from build123d import *

# Parameters (mm, degrees)
SKETCH1_R         = 9.5
SKETCH1_R_2       = 8
EXTRUDE1_DEPTH    = 1.5
SKETCH2_R         = 10.5
SKETCH2_R_2       = 8
EXTRUDE2_DEPTH    = 1.5
EXTRUDE3_START    = 6.5
SKETCH3_R         = 9.5
EXTRUDE3_DEPTH    = 6.5
EXTRUDE4_START    = 1.5
SKETCH4_R         = 9.5
SKETCH4_R_2       = 5
EXTRUDE4_DEPTH    = 1.5
SKETCH5_R         = 5
EXTRUDE5_DEPTH    = 19.479718613
SKETCH6_R         = 0.75
EXTRUDE6_DEPTH    = 18.628102564
CIRPATTERN1_COUNT = 4
EXTRUDE7_START    = 10
SKETCH7_R         = 6.5
SKETCH7_R_2       = 5
EXTRUDE7_DEPTH    = 10
SKETCH8_R         = 6.5
SKETCH8_W         = 5
SKETCH8_H         = 5
EXTRUDE8_DEPTH    = 1.5


with BuildPart() as part:
    # Sketch1 → Extrude1 (new body)
    with BuildSketch(Plane.XY):
        Circle(SKETCH1_R)
        Circle(SKETCH1_R_2, mode=Mode.SUBTRACT)
    extrude(amount=EXTRUDE1_DEPTH)

    # Sketch2 → Extrude2 (add)
    with BuildSketch(Plane.XY.offset(1.5)):
        Circle(SKETCH2_R)
        Circle(SKETCH2_R_2, mode=Mode.SUBTRACT)
    extrude(amount=EXTRUDE2_DEPTH)

    # Sketch3 → Extrude3 (add)
    with BuildSketch(Plane(origin=(0, 0, 0), x_dir=(-1, 0, 0), z_dir=(0, 0, -1)).offset(EXTRUDE3_START)):
        Circle(SKETCH3_R)
        with BuildLine():
            Line((-7.332121112, 3.2), (-3.2, 3.2))
            Line((-3.2, 3.2), (-3.2, 7.332121112))
            ThreePointArc((-3.2, 7.332121112), (0, 8), (3.2, 7.332121112))
            Line((3.2, 7.332121112), (3.2, 3.2))
            Line((3.2, 3.2), (7.332121112, 3.2))
            ThreePointArc((7.332121112, 3.2), (8, 0), (7.332121112, -3.2))
            Line((7.332121112, -3.2), (3.2, -3.2))
            Line((3.2, -3.2), (3.2, -7.332121112))
            ThreePointArc((3.2, -7.332121112), (0, -8), (-3.2, -7.332121112))
            Line((-3.2, -7.332121112), (-3.2, -3.2))
            Line((-3.2, -3.2), (-7.332121112, -3.2))
            ThreePointArc((-7.332121112, -3.2), (-8, 0), (-7.332121112, 3.2))
        make_face(mode=Mode.SUBTRACT)
    extrude(amount=-EXTRUDE3_DEPTH)

    # Sketch4 → Extrude4 (add)
    with BuildSketch(Plane(origin=(0, 0, -6.5), x_dir=(-1, 0, 0), z_dir=(0, 0, -1)).offset(EXTRUDE4_START)):
        Circle(SKETCH4_R)
        with Locations(Location((0, 0, 0), (0, 0, 140.2081805))):
            Circle(SKETCH4_R_2, mode=Mode.SUBTRACT)
    extrude(amount=-EXTRUDE4_DEPTH)

    # Sketch5 → Extrude5 (cut, through all)
    with BuildSketch(Plane(origin=(0, 0, -8), x_dir=(-1, 0, 0), z_dir=(0, 0, -1))):
        with Locations(Location((0, 0, 0), (0, 0, 140.2081805))):
            Circle(SKETCH5_R)
    extrude(amount=-EXTRUDE5_DEPTH, mode=Mode.SUBTRACT)

    # Sketch6 → Extrude6 (cut, through all)
    with BuildSketch(Plane.XY.offset(-6.5)):
        with Locations((7.03562364, 1.75)):
            Circle(SKETCH6_R)
        with Locations(Location((7.03562364, -1.75, 0), (0, 0, 346.033020145))):
            Circle(SKETCH6_R)
    extrude6 = extrude(amount=-EXTRUDE6_DEPTH, mode=Mode.SUBTRACT)

    # CirPattern1: Extrude6 ×4 about axis
    cirpattern1_axis = Axis((0, 0, 0), (0, 0, 1))
    for i in range(1, CIRPATTERN1_COUNT):
        add(extrude6.rotate(cirpattern1_axis, i * 360 / CIRPATTERN1_COUNT), mode=Mode.SUBTRACT)

    # Sketch7 → Extrude7 (add)
    with BuildSketch(Plane(origin=(0, 0, -8), x_dir=(-1, 0, 0), z_dir=(0, 0, -1)).offset(EXTRUDE7_START)):
        with Locations(Location((0, 0, 0), (0, 0, 193.967860451))):
            Circle(SKETCH7_R)
        with Locations(Location((0, 0, 0), (0, 0, 140.2081805))):
            Circle(SKETCH7_R_2, mode=Mode.SUBTRACT)
    extrude(amount=-EXTRUDE7_DEPTH)

    # Sketch8 → Extrude8 (add)
    with BuildSketch(Plane(origin=(0, 0, -18), x_dir=(-1, 0, 0), z_dir=(0, 0, -1))):
        with Locations(Location((0, 0, 0), (0, 0, 193.967860451))):
            Circle(SKETCH8_R)
        Rectangle(SKETCH8_W, SKETCH8_H, mode=Mode.SUBTRACT)
    extrude(amount=-EXTRUDE8_DEPTH)


solid = part.part
Geometry check sheet. Reference: the model listing, model coordinates, mm. A direction names the side the tool comes from. Give positions to 0.01 mm unless a question says otherwise; leave off trailing zeros. Order: outer loops, then holes, each group sorted by start corner. A loop starts at its lowest first (then second) coordinate and runs counter-clockwise, first axis right, second up. Notation, with made-up numbers: (19, 30) - (25, 30) arc R16 ccw to (25, 51) - close; hole circle Ø9 at (48, 22). An arc over 180 degrees is marked (long way). Use one line per item in the form item = value.
1) Access from +Z, -Z, +X, -X, +Y, -Y to the whole of each face (thin tool, end or side, straight path). Record for faces 1 (the face through (3.2, 6, -3)), 2 (the face through (0, -2.5, -17)), 3 (the face through (-5, -9, 1.5)).
Working result:
face_1 = +Z
face_2 = +Z, -Z
face_3 = -Z
2) Sectioned sample at C-C (z = -7.25). Count the separate pieces of the cut face and the enclosed holes in it, and give its area (3 significant figures).
Working result:
separate_pieces = 1
enclosed_holes = 9
area = 191 mm^2
3) Draft check along Y on faces 4 (the face through (1.783, -6.286, -7.24)), 5 (the face through (-2, -8, 3)). Enter one of: released by +Y, released by -Y, zero draft, split by the parting line, or undercut.
Working result:
face_4 = undercut
face_5 = zero draft
4) Sectioned sample at A-A (x = 0). Record the boundary of the cut face in (y, z), and give its area (3 significant figures).
Working result:
outline = (-10.5, 1.5) - (-9.5, 1.5) - (-9.5, -8) - (-6.5, -8) - (-6.5, -18) - (-2.5, -18) - (-2.5, -16.5) - (-5, -16.5) - (-5, -6.5) - (-8, -6.5) - (-8, 3) - (-10.5, 3) - close; (2.5, -18) - (6.5, -18) - (6.5, -8) - (9.5, -8) - (9.5, 1.5) - (10.5, 1.5) - (10.5, 3) - (8, 3) - (8, -6.5) - (5, -6.5) - (5, -16.5) - (2.5, -16.5) - close
area = 82.5 mm^2
5) Depth check by flat-ended pin: pin 1 Ø1.2 at (y, z) = (0.5, -17) entering from -X; pin 2 Ø2 at (x, z) = (-5, -9.5) entering from +Y; pin 3 Ø3 at (x, z) = (-5, -4) entering from -Y. Enter the tip coordinate at first touch or a pass-through.
Working result:
pin_1 = -6.5
pin_2 = 5.12
pin_3 = -8.83
6) Sectioned sample at D-D (x = 4.5). Record the boundary of the cut face in (y, z).
Working result:
outline = (-9.49, 1.5) - (-8.37, 1.5) - (-8.37, -8) - (-4.69, -8) - (-4.69, -18) - (4.69, -18) - (4.69, -8) - (8.37, -8) - (8.37, 1.5) - (9.49, 1.5) - (9.49, 3) - (6.61, 3) - (6.61, 0) - (3.2, 0) - (3.2, -6.5) - (2.18, -6.5) - (2.18, -16.5) - (-2.18, -16.5) - (-2.18, -6.5) - (-3.2, -6.5) - (-3.2, 0) - (-6.61, 0) - (-6.61, 3) - (-9.49, 3) - close
7) Material ranges on probe 1 along Y at (x, z) = (1.75, -7.3); probe 2 along Z at (x, y) = (3, 8), recorded low to high. Write a range as from..to.
Working result:
probe_1 = -9.34..-7.79, -6.29..-4.68, 4.68..6.29, 7.79..9.34
probe_2 = -8..3
